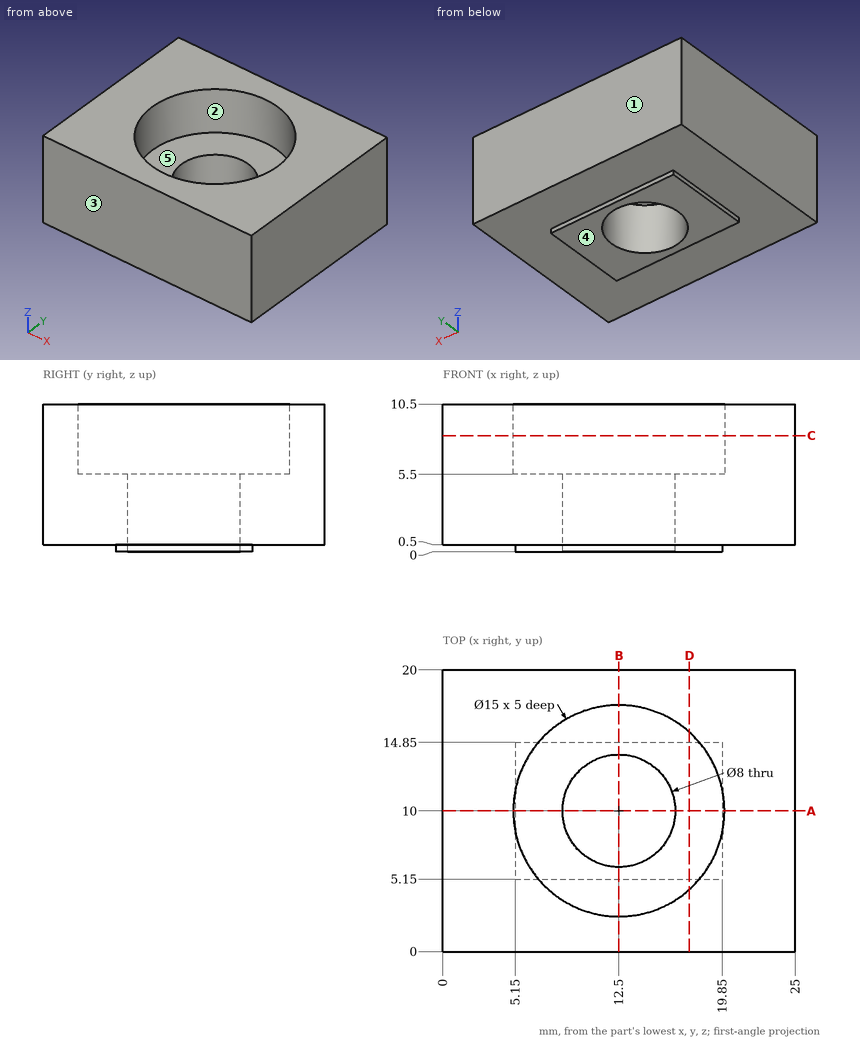
Job drawing, mm, ordinate dimensions from the low corner. One solid piece. A direction names the side the tool comes from. Coordinates: 2 decimals unless noted, no trailing zeros. Order: outer loops, then holes, each group sorted by start corner. A loop starts at its lowest first (then second) coordinate and runs counter-clockwise, first axis right, second up. Notation, with made-up numbers: (25, 63.5) -> (57, 63.5) arc R9 cw to (57, 70.5) -> close; hole circle Ø1 at (43.25, -21). An arc over 180 degrees is marked (long way). Return JSON: item names as keys, results as strings. Group by question number.
Item 1: Tool access for the marked faces 1 and 2: list every direction of +Z, -Z, +X, -X, +Y, -Y with a clear straight run to the whole face (end or side of a thin tool).
Item 2: Saw through at A-A on y = 10. Write the cut outline in (x, z).
Item 3: Saw through at B-B on x = 12.5. Write the cut outline in (y, z), then the cut area to 4 significant figures.
Item 4: Saw through at D-D on x = 17.5. Write the cut outline in (y, z), then the cut area to 3 significant figures.
Item 5: Flat gauge pins, fed straight in: P1, Ø0.6, axis at x = 16, z = 0, coming from the -Y side; P2, Ø4.5, axis at x = 13, y = 9, coming from the +Z side; P3, Ø0.6, axis at y = 12.5, z = 0, coming from the +X side. Where does each tip first touch, or does it go through?
Item 6: Pull direction Y, two halves, no side cores. Call the marked faces 3, 4 and 5: pulls with the +Y half, pulls with the -Y half, needs draft (parallel to the pull), parting line crosses it, or undercut.
Item 7: Saw through at C-C on z = 8.25. Write the cut outline in (x, y).
Item 8: Wall check: line 1 along Y through (x, z) = (12.5, 1.65); line 2 along X through (y, z) = (10, 1.55); line 3 along Z through (x, y) = (10, 3.25). Give the ranges that are in metal, low to high. Write a range as [from, to].
Values found:
{
 "1": {"face 1": "+Z, -Z, +X, -X, +Y", "face 2": "+Z"},
 "2": {"outline": "(0, 0.5) -> (5.15, 0.5) -> (5.15, 0) -> (8.5, 0) -> (8.5, 5.5) -> (5, 5.5) -> (5, 10.5) -> (0, 10.5) -> close; (16.5, 0) -> (19.85, 0) -> (19.85, 0.5) -> (25, 0.5) -> (25, 10.5) -> (20, 10.5) -> (20, 5.5) -> (16.5, 5.5) -> close"},
 "3": {"outline": "(0, 0.5) -> (5.15, 0.5) -> (5.15, 0) -> (6, 0) -> (6, 5.5) -> (2.5, 5.5) -> (2.5, 10.5) -> (0, 10.5) -> close; (14, 0) -> (14.85, 0) -> (14.85, 0.5) -> (20, 0.5) -> (20, 10.5) -> (17.5, 10.5) -> (17.5, 5.5) -> (14, 5.5) -> close", "area": "85.85 mm2"},
 "4": {"outline": "(0, 0.5) -> (5.15, 0.5) -> (5.15, 0) -> (14.85, 0) -> (14.85, 0.5) -> (20, 0.5) -> (20, 10.5) -> (15.59, 10.5) -> (15.59, 5.5) -> (4.41, 5.5) -> (4.41, 10.5) -> (0, 10.5) -> close", "area": "149 mm2"},
 "5": {"P1": "stops at y = 5.15", "P2": "passes through", "P3": "stops at x = 19.85"},
 "6": {"face 3": "pulls with the -Y half", "face 4": "needs draft", "face 5": "undercut"},
 "7": {"outline": "(0, 0) -> (25, 0) -> (25, 20) -> (0, 20) -> close; hole circle Ø15 at (12.5, 10)"},
 "8": {"line 1": "y = [0, 6], [14, 20]", "line 2": "x = [0, 8.5], [16.5, 25]", "line 3": "z = [0.5, 5.5]"}
}
